Geometry check sheet. Reference: the model listing, model coordinates, mm. Face numbers are marked on the shaded views. Round coordinates to 2 decimals unless told otherwise and drop trailing zeros. Write each loop counter-clockwise with the first axis right and the second up, starting at its lowest first coordinate (ties: lowest second). Pieces come first, ordered by that corner, then holes. Notation, with made-up numbers: (-26.5, -21.75) - (-17.5, -21.75) arc R9 cw to (-17.5, -16.75) - close; hole circle Ø6 at (35, 28.5). An arc over 180 degrees is marked (long way). Return JSON: item names as keys, results as strings.
```python
from build123d import *

# Parameters (mm, degrees)
F1_DEPTH = 56.5685424949
F5_DEPTH = 5
F6_DEPTH = 25


with BuildPart() as f1:
    # F0 (on Top) → F1 (new body)
    with BuildSketch(Plane.XY):
        Polygon((20, -20), (20, 20), (-20, 20), align=None)
    extrude(amount=F1_DEPTH)

    # F4 (on face) → F5 (join, symmetric)
    with BuildSketch(Plane(origin=(10, -10, 14.1421356237), x_dir=(0.8660254038, 0.2886751346, -0.4082482905), z_dir=(-0.5, 0.5, -0.7071067812))):
        Polygon((-28.3771324027, -29.5247237874), (-28.3771324027, -40.1313255052), (-20.8771324027, -29.5247237874), align=None)
        Polygon((-4.7168783649, 3.9359283621), (-4.7168783649, -6.6706733557), (2.7831216351, 3.9359283621), align=None)
    extrude(amount=F5_DEPTH, both=True)

    # F4 (on face) → F6 (join, symmetric)
    with BuildSketch(Plane(origin=(10, -10, 14.1421356237), x_dir=(0.8660254038, 0.2886751346, -0.4082482905), z_dir=(-0.5, 0.5, -0.7071067812))):
        Polygon((-16.5470053838, -12.7943977126), (-16.5470053838, -23.4009994304), (-11.5470053838, -16.3299316186), align=None)
        Polygon((-9.0470053838, -12.7943977126), (-16.5470053838, -12.7943977126), (-11.5470053838, -16.3299316186), align=None)
    extrude(amount=F6_DEPTH, both=True)


solid = f1.part
```
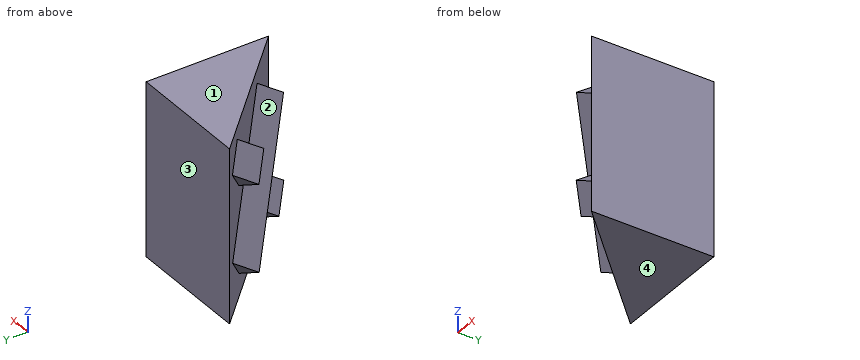
(1) Section check B-B, the plane y = 0. Enter the section's corners in (x, z), plus the area to 3 significant figures.
Response values:
{"outline": "(-8.66, 22.16) - (0, 22.16) - (0, 0) - (20, 0) - (20, 56.57) - (0, 56.57) - (0, 40.53) - close", "area": "1,210 mm^2"}
(2) Material ranges on line 1 along X through (y, z) = (0, 41.5); line 2 along Z through (x, y) = (-15, 13); line 3 along Z through (x, y) = (9, -15), recorded low to high. Write a range as [from, to].
Response values:
{"line 1": "x = [0, 20]", "line 2": "z = [12.73, 17.9], [41.01, 46.88]", "line 3": "z = [14.4, 18.38], [43.37, 46.67]"}
(3) Release check for a two-part mould opening along Z. For the marked faces 1, 2, 3 and 4 record: pulls with the +Z half, pulls with the -Z half, needs draft (parallel to the pull), parting line crosses it, or undercut.
Response values:
{"face 1": "pulls with the +Z half", "face 2": "undercut", "face 3": "needs draft", "face 4": "pulls with the -Z half"}
(4) Section check A-A, the plane x = -3. Enter the section's corners in (y, z), plus the area to 3 significant figures.
Response values:
{"outline": "(-5.66, 30.17) - (3, 17.92) - (3, 0) - (20, 0) - (20, 56.57) - (3, 56.57) - (3, 36.29) - close", "area": "1,040 mm^2"}
(5) Section check C-C, the plane z = 48. Enter the section's corners in (x, y).
Response values:
{"outline": "(-20, 20) - (-15.21, 15.21) - (-12.08, 5.81) - (-8.94, 8.94) - (5.28, -5.28) - (8.17, -13.95) - (11.06, -11.06) - (20, -20) - (20, 20) - close"}
(6) Gauge pin test, flat ends, axial feed: pin 1 (5 mm diameter, centred on x = 10.5, y = -4, fed in from -Z); pin 2 (12 mm diameter, centred on x = -14.5, y = 2.5, fed in from -Z); pin 3 (8 mm diameter, centred on x = 9.5, z = 42, fed in from -Y). Record the tip position at first contact, or that the pin passes through.
Response values:
{"pin 1": "stops at z = 0", "pin 2": "stops at z = 10.14", "pin 3": "stops at y = -16.75"}
(7) Section check D-D, the plane x = 5. Enter the section's corners in (y, z), plus the area to 3 significant figures.
Response values:
{"outline": "(-13.66, 12.5) - (-11.55, 9.51) - (-5, 14.14) - (-5, 0) - (20, 0) - (20, 56.57) - (-5, 56.57) - (-5, 47.6) - (-13.66, 41.48) - (-5, 29.23) - (-5, 18.63) - close", "area": "1,530 mm^2"}
